Design review of the part built by this model. Coordinates are the model's own, in mm. Face numbers are marked on the shaded views. A direction names the side the tool comes from. Coordinates: 2 decimals unless noted, no trailing zeros. Write each loop counter-clockwise with the first axis right and the second up, starting at its lowest first coordinate (ties: lowest second). Pieces come first, ordered by that corner, then holes. Notation, with made-up numbers: (35.25, 60) -> (92.25, 60) arc R27 ccw to (92.25, 76) -> close; hole circle Ø2 at (5.5, -22). An arc over 180 degrees is marked (long way). Answer in a Markdown table with one row per item. Add a question column.
Item 1: Clearance check with flat-ended pins moving along their axes: P1, Ø6, axis at x = -99.5, z = 4.5, coming from the +Y side; P2, Ø1.5, axis at x = -94.5, z = 9, coming from the -Y side; P3, Ø4, axis at x = -104, y = -49, coming from the +Z side. State where each tip first meets the part, or that it passes through.
Item 2: Take a section at B-B, the plane y = -45. Write out the cut boundary in (x, z), and give its area (3 significant figures).
Item 3: Take a section at A-A, the plane z = -13.5. Write out the cut boundary in (x, y).
Item 4: For the marked faces 1, 2, 3, 4 and 5, list the 3-axis set-ups (+Z, -Z, +X, -X, +Y, -Y) from which the entire face can be reached by the end or side of a thin tool; tool diameter is ignored.
Item 5: To check wall thickness, follow line 1 (Y direction, x = -92.8, z = -13.5); line 2 (Y direction, x = -100.5, z = 6); line 3 (X direction, y = -33.25, z = 7). State the ranges of each line that lie inside material, in increasing order.
Item 6: Take a section at D-D, the plane y = -41.5. Write out the cut boundary in (x, z).
Item 7: Take a section at C-C, the plane z = -2. Write out the cut boundary in (x, y).
from build123d import *

# Parameters (mm, degrees)
PLATE_START              = -91.6
PLATE_SKETCH_W           = 34
PLATE_SKETCH_H           = 30
PLATE_SKETCH_R           = 1.7
PLATE_DEPTH              = 1.6
MATEK_START              = -93.2
MATEK_M10Q_5883_SKETCH_W = 20
MATEK_M10Q_5883_SKETCH_H = 20
MATEK_M10Q_5883_DEPTH    = 12.4


with BuildPart() as part:
    # Plate Sketch → Plate (new body)
    with BuildSketch(Plane(origin=(0, 0, 0), x_dir=(0, 0, -1), z_dir=(1, 0, 0)).offset(PLATE_START)):
        with Locations((0, -45)):
            Rectangle(PLATE_SKETCH_W, PLATE_SKETCH_H)
        with Locations((13.5, -45)):
            Circle(PLATE_SKETCH_R, mode=Mode.SUBTRACT)
        with Locations((-13.5, -45)):
            Circle(PLATE_SKETCH_R, mode=Mode.SUBTRACT)
    extrude(amount=-PLATE_DEPTH)

    # Matek M10Q-5883 Sketch → Matek M10Q-5883 (add)
    with BuildSketch(Plane(origin=(0, 0, 0), x_dir=(0, 0, -1), z_dir=(1, 0, 0)).offset(MATEK_START)):
        with Locations((0, -45)):
            Rectangle(MATEK_M10Q_5883_SKETCH_W, MATEK_M10Q_5883_SKETCH_H)
    extrude(amount=-MATEK_M10Q_5883_DEPTH)


solid = part.part
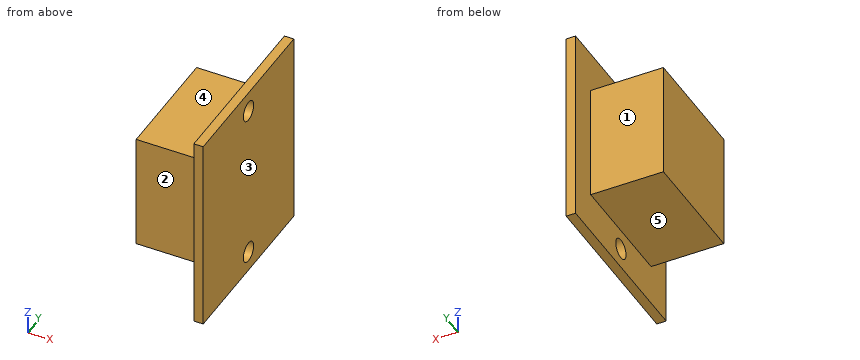
Answers:
| question | item | result |
|---|---|---|
| 1 | P1 | stops at y = -35 |
| 1 | P2 | stops at y = -55 |
| 1 | P3 | stops at z = 10 |
| 2 | outline | (-105.6, -10) -> (-93.2, -10) -> (-93.2, -11.8) -> (-91.6, -11.8) -> (-91.6, 11.8) -> (-93.2, 11.8) -> (-93.2, 10) -> (-105.6, 10) -> close; (-93.2, -17) -> (-91.6, -17) -> (-91.6, -15.2) -> (-93.2, -15.2) -> close; (-93.2, 15.2) -> (-91.6, 15.2) -> (-91.6, 17) -> (-93.2, 17) -> close |
| 2 | area | 292 mm^2 |
| 3 | outline | (-93.2, -60) -> (-91.6, -60) -> (-91.6, -46.7) -> (-93.2, -46.7) -> close; (-93.2, -43.3) -> (-91.6, -43.3) -> (-91.6, -30) -> (-93.2, -30) -> close |
| 4 | face 1 | +Z, -Z, -X, +Y |
| 4 | face 2 | +Z, -Z, -X, -Y |
| 4 | face 3 | +Z, -Z, +X, +Y, -Y |
| 4 | face 4 | +Z, -X, +Y, -Y |
| 4 | face 5 | -Z, -X, +Y, -Y |
| 5 | line 1 | y = -60 to -46.7, -43.3 to -30 |
| 5 | line 2 | y = -55 to -35 |
| 5 | line 3 | x = -93.2 to -91.6 |
| 6 | outline | (-105.6, -10) -> (-93.2, -10) -> (-93.2, -17) -> (-91.6, -17) -> (-91.6, 17) -> (-93.2, 17) -> (-93.2, 10) -> (-105.6, 10) -> close |
| 7 | outline | (-105.6, -55) -> (-93.2, -55) -> (-93.2, -60) -> (-91.6, -60) -> (-91.6, -30) -> (-93.2, -30) -> (-93.2, -35) -> (-105.6, -35) -> close |
